Input: dimensioned drawing with shaded views. Units: mm. Origin: part minimum x, y, z. Coordinates: 2 decimals unless noted, no trailing zeros. Order: outer loops, then holes, each group sorted by start corner. A loop starts at its lowest first (then second) coordinate and runs counter-clockwise, first axis right, second up.
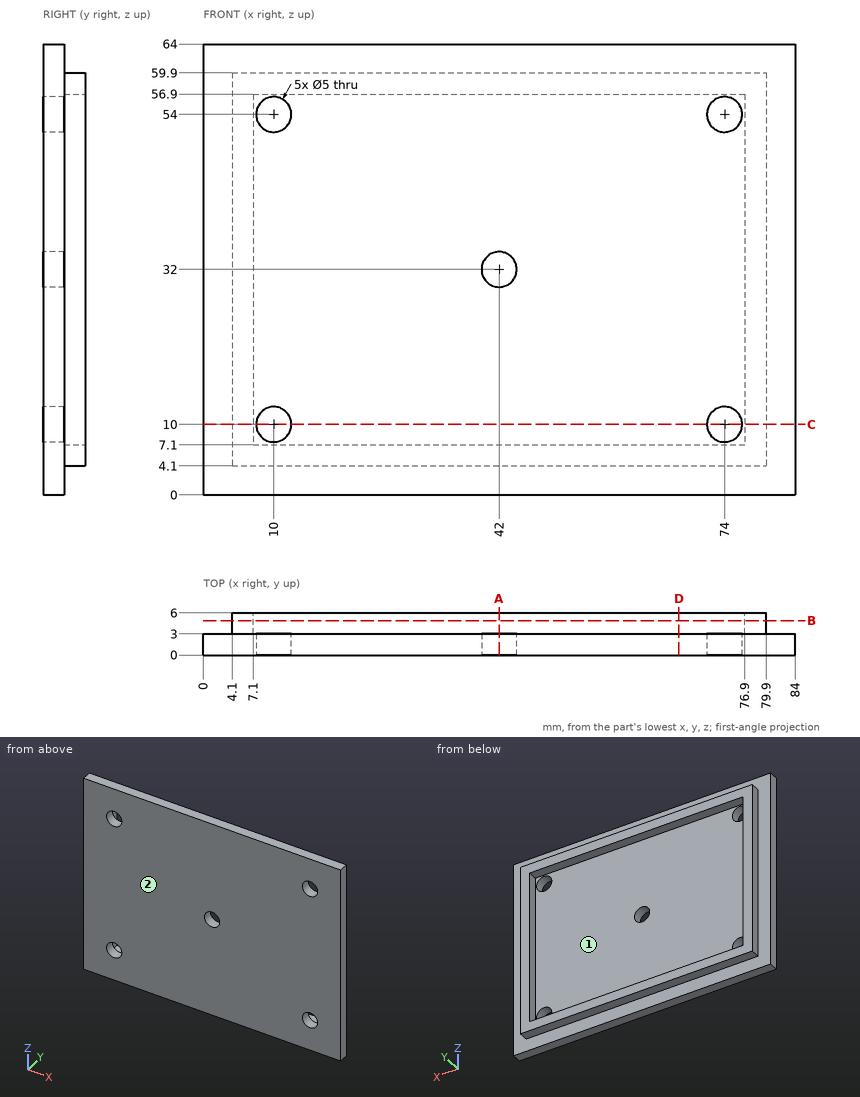
1. Section query D-D, the plane x = 67.5. Output: boundary loops of the cut face in (y, z), plus the area to 3 significant figures.
2. Section query A-A, the plane x = 42. Output: boundary loops of the cut face in (y, z).
3. Material intervals for line 1 along Z through (x, y) = (10, 1.6); line 2 along X through (y, z) = (4.15, 14); line 3 along Z through (x, y) = (42, 0.7), sorted ascending.
4. Contact query for flat-ended pins moving along their axis: P1, Ø0.9, axis at x = 56, y = 4.5, coming from the -Z side; P2, Ø1.5, axis at x = 43, y = 4, coming from the +Z side; P3, Ø2.5, axis at x = 36, y = 4, coming from the +Z side; P4, Ø2.5, axis at y = 4.5, z = 44, coming from the -X side. Output: stop coordinate, or through.
5. Section query C-C, the plane z = 10. Output: boundary loops of the cut face in (x, y).
6. Draft query along X for the marked faces 1 and 2. Return one class per face: +X half, -X half, draft (parallel to the pull), parting line (faces both ways), or undercut.
7. Section query B-B, the plane y = 4.9. Output: boundary loops of the cut face in (x, z), plus the area to 3 significant figures.
Answer key:
1. outline: (0, 0) - (3, 0) - (3, 4.1) - (6, 4.1) - (6, 7.1) - (3, 7.1) - (3, 56.9) - (6, 56.9) - (6, 59.9) - (3, 59.9) - (3, 64) - (0, 64) - close
1. area: 210 mm2
2. outline: (0, 0) - (3, 0) - (3, 4.1) - (6, 4.1) - (6, 7.1) - (3, 7.1) - (3, 29.5) - (0, 29.5) - close; (0, 34.5) - (3, 34.5) - (3, 56.9) - (6, 56.9) - (6, 59.9) - (3, 59.9) - (3, 64) - (0, 64) - close
3. line 1: z = 0 to 7.5, 12.5 to 51.5, 56.5 to 64
3. line 2: x = 4.1 to 7.1, 76.9 to 79.9
3. line 3: z = 0 to 29.5, 34.5 to 64
4. P1: stops at z = 4.1
4. P2: stops at z = 59.9
4. P3: stops at z = 64
4. P4: stops at x = 4.1
5. outline: (0, 0) - (7.5, 0) - (7.5, 3) - (7.1, 3) - (7.1, 6) - (4.1, 6) - (4.1, 3) - (0, 3) - close; (12.5, 0) - (71.5, 0) - (71.5, 3) - (12.5, 3) - close; (76.5, 0) - (84, 0) - (84, 3) - (79.9, 3) - (79.9, 6) - (76.9, 6) - (76.9, 3) - (76.5, 3) - close
6. face 1: undercut
6. face 2: draft
7. outline: (4.1, 4.1) - (79.9, 4.1) - (79.9, 59.9) - (4.1, 59.9) - close; hole (7.1, 7.1) - (76.9, 7.1) - (76.9, 56.9) - (7.1, 56.9) - close
7. area: 754 mm2
